from build123d import *

# Parameters (mm, degrees)
SKETCH1_R           = 77.6224
SKETCH1_R_2         = 76.2
BOSS_EXTRUDE1_DEPTH = 508
SKETCH3_W           = 4.7498
SKETCH3_H           = 203.2
CUT_EXTRUDE1_DEPTH  = 520.72538322
CIRPATTERN2_COUNT   = 4


with BuildPart() as part:
    # Sketch1 → Boss-Extrude1 (new, symmetric)
    with BuildSketch(Plane(origin=(0, 0, 0), x_dir=(1, 0, 0), z_dir=(0, 1, 0))):
        with Locations(Location((0, 0, 0), (0, 0, 270))):
            Circle(SKETCH1_R)
        with Locations(Location((0, 0, 0), (0, 0, 270))):
            Circle(SKETCH1_R_2, mode=Mode.SUBTRACT)
    extrude(amount=BOSS_EXTRUDE1_DEPTH, both=True)

    # Sketch3 → Cut-Extrude1 (cut, through all)
    with BuildSketch(Plane.XY):
        with Locations((0, -330.2)):
            Rectangle(SKETCH3_W, SKETCH3_H)
    cut_extrude1 = extrude(amount=-CUT_EXTRUDE1_DEPTH, mode=Mode.SUBTRACT)

    # CirPattern2: Cut-Extrude1 ×4 about axis
    cirpattern2_axis = Axis((0, 0, 0), (0, 1, 0))
    for i in range(1, CIRPATTERN2_COUNT):
        add(cut_extrude1.rotate(cirpattern2_axis, i * 360 / CIRPATTERN2_COUNT), mode=Mode.SUBTRACT)


solid = part.part
Design review of the part built by this model. Coordinates are the model's own, in mm. Give positions to 0.01 mm unless a question says otherwise; leave off trailing zeros. Order: outer loops, then holes, each group sorted by start corner. A loop starts at its lowest first (then second) coordinate and runs counter-clockwise, first axis right, second up. Notation, with made-up numbers: (71.5, -22) - (122.5, -22) arc R24 cw to (122.5, 4) - close; hole circle Ø3 at (-3, 31.5). An arc over 180 degrees is marked (long way). Write item = value, one per line. Start each with the question number.
Q1. We need section A-A on z = -22. State the section outline as (x, y) points.
Q2. We need section C-C on y = -185. State the section outline as (x, z) points.
Q3. We need section B-B on x = -16. State the section outline as (y, z) points.
Q4. To check wall thickness, follow L1, parallel to Z at x = 0, y = 230; L2, parallel to X at y = 395, z = 58.5. State the ranges of each line that lie inside material, in increasing order. Write a range as from..to.
Q5. Mouldability with a two-part tool opening along Z and no side actions: class faces 1 (the face through (-51, 508, 57)), 2 (the face through (-46.367, -7.112, -60.47)), 3 (the face through (23.316, 7.112, 74.038)) as released by +Z, released by -Z, zero draft, split by the parting line, or undercut.
Q6. Clearance check with flat-ended pins moving along their axes: pin 1 Ø10 at (x, y) = (-16.5, -271.5) entering from +Z; pin 2 Ø1 at (y, z) = (140, 59) entering from +X; pin 3 Ø8 at (y, z) = (-240, -20.5) entering from -X. State where each tip first meets the part, or that it passes through.
Working result:
q1.outline = (-74.44, -508) - (-72.96, -508) - (-72.96, 508) - (-74.44, 508) - close; (72.96, -508) - (74.44, -508) - (74.44, 508) - (72.96, 508) - close
q2.outline = circle Ø155.24 at (0, 0); hole circle Ø152.4 at (0, 0)
q3.outline = (-508, -75.96) - (508, -75.96) - (508, -74.5) - (-508, -74.5) - close; (-508, 74.5) - (508, 74.5) - (508, 75.96) - (-508, 75.96) - close
q4.L1 = -77.62..-76.2, 76.2..77.62
q4.L2 = -51.02..-48.83, 48.83..51.02
q5.face_1 = zero draft
q5.face_2 = undercut
q5.face_3 = split by the parting line
q6.pin_1 = 76.77
q6.pin_2 = 51.02
q6.pin_3 = -75.85
